Here's the drawing with two shaded views (mm, measured from the low corner). I have some questions. A direction names the side the tool comes from. Round coordinates to 2 decimals unless told otherwise and drop trailing zeros. Order: outer loops, then holes, each group sorted by start corner. A loop starts at its lowest first (then second) coordinate and runs counter-clockwise, first axis right, second up. Notation, with made-up numbers: (49, 56) - (67, 56) arc R14 ccw to (67, 64) - close; hole circle Ø5 at (77, 71.5). An arc over 180 degrees is marked (long way). One line per item, written item: value.
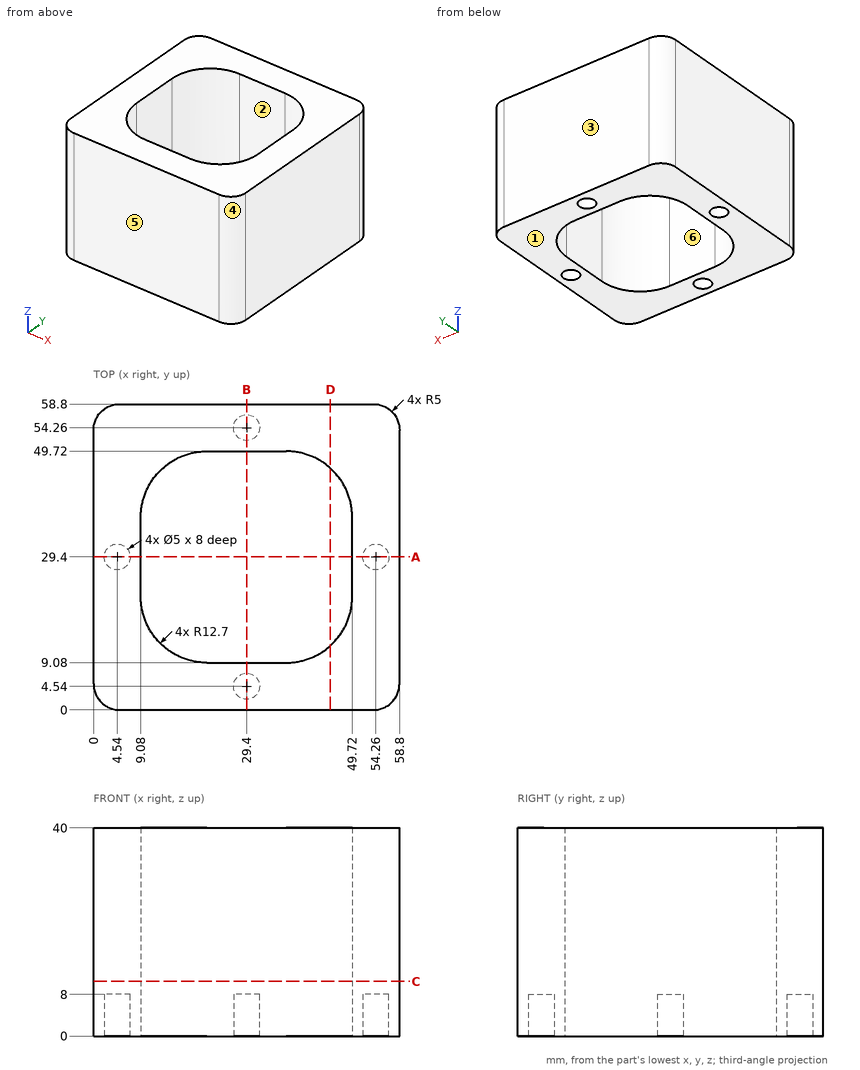
Q1. Which directions (+Z, -Z, +X, -X, +Y, -Y) give clear straight access to the entire face, cutting with the end or side of a thin tool? Please do the marked faces 5 and 6.
Results list:
face 5: +Z, -Z, +X, -X, -Y
face 6: +Z, -Z
Q2. If I drill on line 1 along X through (y, z) = (29.4, 2.25); line 2 along X through (y, z) = (54, 3), over which ranges is the centre line in solid material (lowest first)?
Results list:
line 1: 0 to 2.04, 7.04 to 9.08, 49.72 to 51.76, 56.76 to 58.8
line 2: 0 to 26.91, 31.89 to 58.8
Q3. If we section it at D-D, the plane x = 45.5: Please give me the cut outline in (y, z), then the cut area to 3 significant figures.
Results list:
outline: (0, 0) - (12.33, 0) - (12.33, 40) - (0, 40) - close; (46.47, 0) - (58.8, 0) - (58.8, 40) - (46.47, 40) - close
area: 986 mm²
Q4. If we section it at C-C, the plane z = 10.5: Please give me the cut outline in (x, y), then the cut area to 3 significant figures.
Results list:
outline: (0, 5) arc R5 ccw to (5, 0) - (53.8, 0) arc R5 ccw to (58.8, 5) - (58.8, 53.8) arc R5 ccw to (53.8, 58.8) - (5, 58.8) arc R5 ccw to (0, 53.8) - close; hole (9.08, 21.78) arc R12.7 ccw to (21.78, 9.08) - (37.02, 9.08) arc R12.7 ccw to (49.72, 21.78) - (49.72, 37.02) arc R12.7 ccw to (37.02, 49.72) - (21.78, 49.72) arc R12.7 ccw to (9.08, 37.02) - close
area: 1,920 mm²
Q5. We'd pull the mould along Y, two halves only. Please class the marked faces 1, 2, 3 and 4: released by +Y, released by -Y, zero draft, split by the parting line, or undercut.
Results list:
face 1: zero draft
face 2: undercut
face 3: released by +Y
face 4: released by -Y
Q6. If we section it at A-A, the plane y = 29.4: Please give me the cut outline in (x, z).
Results list:
outline: (0, 0) - (2.04, 0) - (2.04, 8) - (7.04, 8) - (7.04, 0) - (9.08, 0) - (9.08, 40) - (0, 40) - close; (49.72, 0) - (51.76, 0) - (51.76, 8) - (56.76, 8) - (56.76, 0) - (58.8, 0) - (58.8, 40) - (49.72, 40) - close
Q7. Will these pins go through, and if not, where does the flat tip stop? pin 1 (4 mm diameter, centred on x = 4.5, y = 29.5, fed in from -Z); pin 2 (10 mm diameter, centred on x = 19.5, y = 40.5, fed in from -Z).
Results list:
pin 1: z = 8
pin 2: through
